Design review of the part shown in the three views and the two pictorial views. Dimensions are in mm from the part's minimum x, y and z. Round coordinates to 2 decimals unless told otherwise and drop trailing zeros. Loops run counter-clockwise (first coordinate to the right, second up) from the corner with the lowest first, then second, coordinate; pieces in that order, holes last. Notation, with made-up numbers: M 71.25,14 L 84.25,14 A18 ccw 84.25,30 Z; hole C -23,-12 d4. An arc over 180 degrees is marked long. One line per question, with ' | ' between items. Start each with the question number.
1) We need section A-A (z = 6.5). Give the boundary of the cut face in (x, y), and give its area (3 significant figures).
2) For probe 1 along X at (y, z) = (36, 6.25); probe 2 along Z at (x, y) = (76.5, 35); probe 3 along Y at (x, z) = (78, 3.75), list the stretches that pass through material, from the lowest coordinate up. Write a range as from..to.
3) For pin 1 Ø2 at (y, z) = (2, 3) entering from +X; pin 2 Ø2.5 at (x, z) = (155, 5.5) entering from -Y; pin 3 Ø2 at (y, z) = (35.5, 2) entering from -X, all flat-tipped, find the tip position at first contact; note any pin that passes through.
4) Mouldability with a two-part tool opening along Z and no side actions: class the marked faces 1 and 2 as pulls with the +Z half, pulls with the -Z half, needs draft (parallel to the pull), parting line crosses it, or undercut.
5) We need section B-B (x = 104.5). Give the boundary of the cut face in (y, z).
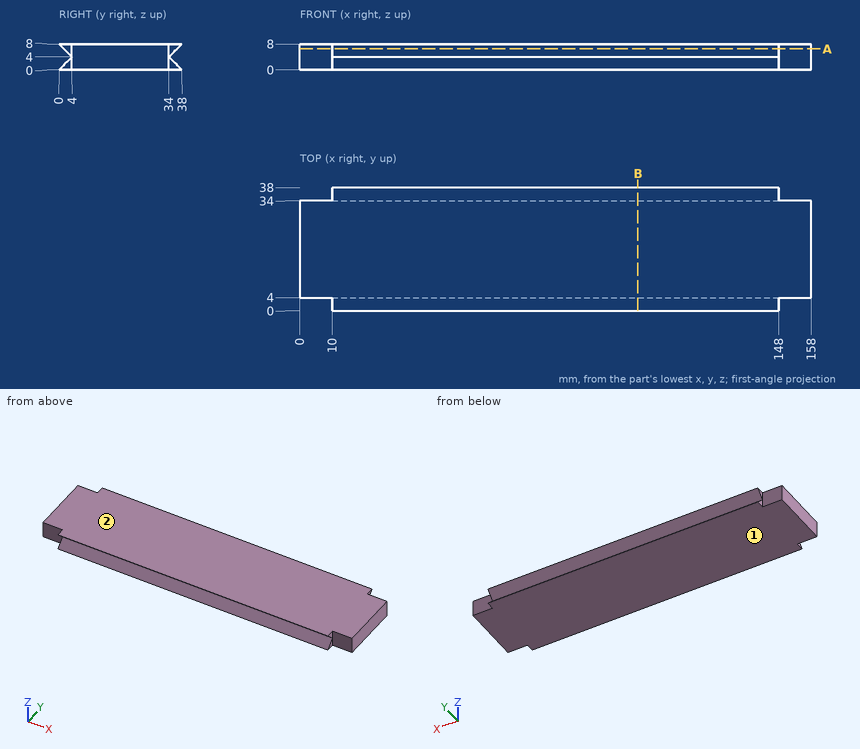
Answers below:
1) outline: M 0,4 L 10,4 L 10,1.5 L 148,1.5 L 148,4 L 158,4 L 158,34 L 148,34 L 148,36.5 L 10,36.5 L 10,34 L 0,34 Z | area: 5,430 mm^2
2) probe 1: 10..148 | probe 2: 0..3, 5..8 | probe 3: 3.75..34.25
3) pin 1: x = 148 | pin 2: y = 4 | pin 3: x = 10
4) face 1: pulls with the -Z half | face 2: pulls with the +Z half
5) outline: M 0,0 L 38,0 L 34,4 L 38,8 L 0,8 L 4,4 Z
